Read the model definition and answer for the solid it produces. Units are mm, in the model's axes. Give positions to 0.01 mm unless a question says otherwise; leave off trailing zeros. Write each loop counter-clockwise with the first axis right and the second up, starting at its lowest first coordinate (ties: lowest second). Pieces come first, ordered by that corner, then holes. Notation, with made-up numbers: (49, 76) -> (68, 76) arc R6 cw to (68, 81) -> close; hole circle Ø8 at (55.5, 19.25). An arc over 180 degrees is marked (long way). Answer as CSV lines item,"result". Start each with the question number.
1. Find the intervals of material crossed by line 1 (Y direction, x = 130, z = 1.4); line 2 (Y direction, x = 60, z = 3.4); line 3 (X direction, y = 100, z = 4.4), in increasing order.
2. The part is cut by section D-D, the plane x = 135. Determine the outline of the cut face in (y, z).
3. For a pull along X with two mould halves and no side action, classify faces 1 (the flat face through (74, 110, 3)), 2 (the flat face through (150, 54, 3)), 3 (the cylindrical face through (86.908, 10.601, 3.042)) as pulls with the +X half, pulls with the -X half, needs draft (parallel to the pull), parting line crosses it, or undercut.
4. The part is cut by section C-C, the plane y = 90. Determine the outline of the cut face in (x, z), and give its area (3 significant figures).
5. The part is cut by section B-B, the plane y = 10. Determine the outline of the cut face in (x, z).
6. The part is cut by section A-A, the plane x = 110. Determine the outline of the cut face in (y, z).
from build123d import *

# Parameters (mm, degrees)
ESQUISSE1_W             = 150
ESQUISSE1_H             = 110
BOSS_EXTRU_1_DEPTH      = 6
ESQUISSE2_R             = 2
ENL_V_MAT_EXTRU_1_DEPTH = 187.107495819
ESQUISSE3_R             = 7
ENL_V_MAT_EXTRU_2_DEPTH = 187.107495819
ESQUISSE4_R             = 1.5
ENL_V_MAT_EXTRU_3_DEPTH = 6


with BuildPart() as part:
    # Esquisse1 → Boss.-Extru.1 (new body)
    with BuildSketch(Plane.XY):
        with Locations((75, 55)):
            Rectangle(ESQUISSE1_W, ESQUISSE1_H)
    extrude(amount=BOSS_EXTRU_1_DEPTH)

    # Esquisse2 → Enlèv. mat.-Extru.1 (cut, through all)
    with BuildSketch(Plane.XY.offset(6)):
        with Locations((110, 10)):
            Circle(ESQUISSE2_R)
        with Locations((135, 10)):
            Circle(ESQUISSE2_R)
        with Locations(Location((35, 10, 0), (0, 0, 180))):
            Circle(ESQUISSE2_R)
        with Locations(Location((60, 10, 0), (0, 0, 180))):
            Circle(ESQUISSE2_R)
        with Locations((85, 10)):
            Circle(ESQUISSE2_R)
    extrude(amount=-ENL_V_MAT_EXTRU_1_DEPTH, mode=Mode.SUBTRACT)

    # Esquisse3 → Enlèv. mat.-Extru.2 (cut, through all)
    with BuildSketch(Plane.XY.offset(6)):
        with Locations((130, 90)):
            Circle(ESQUISSE3_R)
    extrude(amount=-ENL_V_MAT_EXTRU_2_DEPTH, mode=Mode.SUBTRACT)

    # Esquisse4 → Enlèv. mat.-Extru.3 (cut)
    with BuildSketch(Plane.XY.offset(6)):
        with Locations((130, 100)):
            Circle(ESQUISSE4_R)
        with Locations((140, 90)):
            Circle(ESQUISSE4_R)
        with Locations((130, 80)):
            Circle(ESQUISSE4_R)
        with Locations((120, 90)):
            Circle(ESQUISSE4_R)
    extrude(amount=-ENL_V_MAT_EXTRU_3_DEPTH, mode=Mode.SUBTRACT)


solid = part.part
Results found:
1,line 1,"y = 0 to 78.5, 81.5 to 83, 97 to 98.5, 101.5 to 110"
1,line 2,"y = 0 to 8, 12 to 110"
1,line 3,"x = 0 to 128.5, 131.5 to 150"
2,outline,"(0, 0) -> (8, 0) -> (8, 6) -> (0, 6) -> close; (12, 0) -> (85.1, 0) -> (85.1, 6) -> (12, 6) -> close; (94.9, 0) -> (110, 0) -> (110, 6) -> (94.9, 6) -> close"
3,face 1,"needs draft"
3,face 2,"pulls with the +X half"
3,face 3,"undercut"
4,outline,"(0, 0) -> (118.5, 0) -> (118.5, 6) -> (0, 6) -> close; (121.5, 0) -> (123, 0) -> (123, 6) -> (121.5, 6) -> close; (137, 0) -> (138.5, 0) -> (138.5, 6) -> (137, 6) -> close; (141.5, 0) -> (150, 0) -> (150, 6) -> (141.5, 6) -> close"
4,area,"780 mm²"
5,outline,"(0, 0) -> (33, 0) -> (33, 6) -> (0, 6) -> close; (37, 0) -> (58, 0) -> (58, 6) -> (37, 6) -> close; (62, 0) -> (83, 0) -> (83, 6) -> (62, 6) -> close; (87, 0) -> (108, 0) -> (108, 6) -> (87, 6) -> close; (112, 0) -> (133, 0) -> (133, 6) -> (112, 6) -> close; (137, 0) -> (150, 0) -> (150, 6) -> (137, 6) -> close"
6,outline,"(0, 0) -> (8, 0) -> (8, 6) -> (0, 6) -> close; (12, 0) -> (110, 0) -> (110, 6) -> (12, 6) -> close"
